from build123d import *

# Parameters (mm, degrees)
SKETCH1_R           = 2.8575
BOSS_EXTRUDE1_DEPTH = 3.5052
CUT_EXTRUDE1_DEPTH  = 1.9558
SKETCH3_R           = 1.7145
BOSS_EXTRUDE2_DEPTH = 22.225


with BuildPart() as part:
    # Sketch1 → Boss-Extrude1 (new body)
    with BuildSketch(Plane(origin=(0, 0, 0), x_dir=(1, 0, 0), z_dir=(0, 1, 0))):
        Circle(SKETCH1_R)
    extrude(amount=BOSS_EXTRUDE1_DEPTH)

    # Sketch2 → Cut-Extrude1 (cut)
    with BuildSketch(Plane.XZ):
        Polygon((1.603951217, 0), (0.801975608, 1.3890625), (-0.801975608, 1.3890625), (-1.603951217, 0), (-0.801975608, -1.3890625), (0.801975608, -1.3890625), align=None)
    extrude(amount=-CUT_EXTRUDE1_DEPTH, mode=Mode.SUBTRACT)

    # Sketch3 → Boss-Extrude2 (add)
    with BuildSketch(Plane(origin=(0, 3.5052, 0), x_dir=(1, 0, 0), z_dir=(0, 1, 0))):
        Circle(SKETCH3_R)
    extrude(amount=BOSS_EXTRUDE2_DEPTH)


solid = part.part
Geometry check sheet. Reference: the model listing, model coordinates, mm. A direction names the side the tool comes from. Give positions to 0.01 mm unless a question says otherwise; leave off trailing zeros. Loops run counter-clockwise (first coordinate to the right, second up) from the corner with the lowest first, then second, coordinate; pieces in that order, holes last.
(1) Release check for a two-part mould opening along Z. For faces 4 (the flat face through (0, 25.73, 0)), 5 (the cylindrical face through (2.726, 1.728, -0.858)), 6 (the flat face through (-1.2, 1, 0.7)) record: released by +Z, released by -Z, zero draft, split by the parting line, or undercut.
From the geometry:
face 4: zero draft
face 5: split by the parting line
face 6: undercut
(2) Section check B-B on z = -0.3. Record the cut outline in (x, y), then the cut area to 3 significant figures.
From the geometry:
outline: (-2.84, 0) - (-1.43, 0) - (-1.43, 1.96) - (1.43, 1.96) - (1.43, 0) - (2.84, 0) - (2.84, 3.51) - (1.69, 3.51) - (1.69, 25.73) - (-1.69, 25.73) - (-1.69, 3.51) - (-2.84, 3.51) - close
area: 89.4 mm2
(3) Section check D-D on z = 2.2. Record the cut outline in (x, y).
From the geometry:
outline: (-1.82, 0) - (1.82, 0) - (1.82, 3.51) - (-1.82, 3.51) - close
(4) Thickness scan on L1, parallel to Y at x = 2.1, z = -0.8; L2, parallel to Z at x = -0.6, y = 19.5; L3, parallel to X at y = 11, z = 0.1. Record the ranges inside material, lowest first.
From the geometry:
L1: y = 0 to 3.51
L2: z = -1.61 to 1.61
L3: x = -1.71 to 1.71
(5) Section check C-C on y = 22. Record the cut outline in (x, z).
From the geometry:
outline: circle Ø3.43 at (0, 0)
(6) Depth check by flat-ended pin: pin 1 Ø3 at (x, y) = (-0.5, 22.5) entering from +Z; pin 2 Ø0.8 at (x, z) = (0, 0) entering from -Y; pin 3 Ø2 at (x, z) = (-1.5, -2) entering from -Y; pin 4 Ø0.5 at (x, y) = (-0.5, 1) entering from -Z. Enter the tip coordinate at first touch or a pass-through.
From the geometry:
pin 1: stops at z = 1.71
pin 2: stops at y = 1.96
pin 3: stops at y = 0
pin 4: stops at z = -2.85
(7) Set-up check for faces 1 (the flat face through (1.2, 0, 1.2)), 2 (the flat face through (0, 1.956, 0)), 3 (the cylindrical face through (-0.372, 14.462, 1.674)): record each of +Z, -Z, +X, -X, +Y, -Y from which the full face is reachable in a straight line by a thin tool's end or side.
From the geometry:
face 1: +Z, -Z, +X, -X, -Y
face 2: -Y
face 3: +Y
(8) Section check A-A on x = 0. Record the cut outline in (y, z), then the cut area to 3 significant figures.
From the geometry:
outline: (0, -2.86) - (3.51, -2.86) - (3.51, -1.71) - (25.73, -1.71) - (25.73, 1.71) - (3.51, 1.71) - (3.51, 2.86) - (0, 2.86) - (0, 1.39) - (1.96, 1.39) - (1.96, -1.39) - (0, -1.39) - close
area: 90.8 mm2
